Part model, mm, in its own coordinate system. Face numbers are marked on the shaded views. Coordinates: 2 decimals unless noted, no trailing zeros. Write each loop counter-clockwise with the first axis right and the second up, starting at its lowest first coordinate (ties: lowest second). Pieces come first, ordered by that corner, then holes. Notation, with made-up numbers: (87.25, -33.5) -> (125.25, -33.5) arc R19 ccw to (125.25, -21.5) -> close; hole circle Ø7 at (53, 82.5). An arc over 180 degrees is marked (long way). One line per question, with ' | ' between items. Start each with the question number.
Item 1: Probe probe 1 along Z at (x, y) = (0, -26.7); probe 2 along X at (y, z) = (-1, 11); probe 3 along Y at (x, z) = (0, 30). List the from-to ranges inside material, lowest first. Write a range as [from, to].
Item 2: Saw through at B-B (y = 20.5). List the corners of the cut face in (x, z).
Item 3: Two-plate mould, pull along Y, no slides. Class the marked faces 1 and 2: pulls with the +Y half, pulls with the -Y half, needs draft (parallel to the pull), parting line crosses it, or undercut.
Item 4: Pin check, flat tips, straight feed: pin 1 (12 mm diameter, centred on y = 14.5, z = 63.5, fed in from -X); pin 2 (6 mm diameter, centred on x = 0, z = 60, fed in from +Y); pin 3 (8 mm diameter, centred on y = -8.5, z = 54, fed in from +X); pin 4 (3 mm diameter, centred on y = 2.5, z = 70.5, fed in from +X). Stop position of each tip, or through.
Item 5: Saw through at A-A (x = 0). List the corners of the cut face in (y, z).
Item 6: Saw through at C-C (x = 18). List the corners of the cut face in (y, z), and give its area (3 significant figures).
Item 7: Saw through at D-D (z = 44). List the corners of the cut face in (x, y).
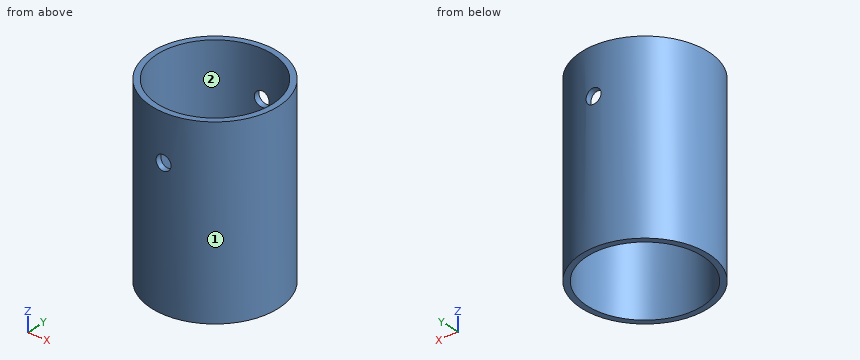
from build123d import *

# Parameters (mm, degrees)
F0_R     = 27.75
F1_DEPTH = 80
F2_T     = -2.5
F3_R     = 3.25
F4_DEPTH = 30


with BuildPart() as f1:
    # F0 (on Top) → F1 (new body)
    with BuildSketch(Plane.XY):
        Circle(F0_R)
    extrude(amount=F1_DEPTH)

    # F2
    f2_openings = [f1.faces().sort_by_distance(p)[0] for p in [
        (0, 0, 80),
        (0, 0, 0),
    ]]
    offset(amount=F2_T, openings=f2_openings)

    # F3 (on Front) → F4 (cut, symmetric)
    with BuildSketch(Plane.XZ):
        with Locations((0, 60)):
            Circle(F3_R)
    extrude(amount=F4_DEPTH, both=True, mode=Mode.SUBTRACT)


solid = f1.part
From the geometry:
1) probe 1: [0, 56.75], [63.25, 80] | probe 2: [-27.73, -25.23], [25.23, 27.73] | probe 3: [-27.75, -25.25], [25.25, 27.75]
2) outline: (-18.7, 0) -> (-14.74, 0) -> (-14.74, 80) -> (-18.7, 80) -> close; (14.74, 0) -> (18.7, 0) -> (18.7, 80) -> (14.74, 80) -> close
3) face 1: parting line crosses it | face 2: undercut
4) pin 1: x = -26.42 | pin 2: through | pin 3: x = 27.38 | pin 4: x = 27.73
5) outline: (-27.75, 0) -> (-25.25, 0) -> (-25.25, 56.75) -> (-27.75, 56.75) -> close; (-27.75, 63.25) -> (-25.25, 63.25) -> (-25.25, 80) -> (-27.75, 80) -> close; (25.25, 0) -> (27.75, 0) -> (27.75, 56.75) -> (25.25, 56.75) -> close; (25.25, 63.25) -> (27.75, 63.25) -> (27.75, 80) -> (25.25, 80) -> close
6) outline: (-21.12, 0) -> (-17.71, 0) -> (-17.71, 80) -> (-21.12, 80) -> close; (17.71, 0) -> (21.12, 0) -> (21.12, 80) -> (17.71, 80) -> close | area: 546 mm2
7) outline: circle Ø55.5 at (0, 0); hole circle Ø50.5 at (0, 0)
